Here's how the part is built. I have some questions about the finished solid (model axes, mm). A direction names the side the tool comes from. Round coordinates to 2 decimals unless told otherwise and drop trailing zeros. Loops run counter-clockwise (first coordinate to the right, second up) from the corner with the lowest first, then second, coordinate; pieces in that order, holes last. Notation, with made-up numbers: (-13.75, 32) -> (-3.75, 32) arc R37 cw to (-3.75, 71) -> close; hole circle Ø6 at (-16, 8.25). An arc over 180 degrees is marked (long way). One line per item, written item: value. Start each with the question number.
```python
from build123d import *

# Parameters (mm, degrees)
PAD_DEPTH    = 30
SKETCH001_R  = 3
POCKET_DEPTH = 5


with BuildPart() as part:
    # Sketch → Pad (new body)
    with BuildSketch(Plane.XY):
        Polygon((0, 0), (0, 53), (47.1, 53), (47.1, 50), (14, 50), (14, 0), (11, 0), (11, 48), (3, 48), (3, 0), align=None)
    extrude(amount=PAD_DEPTH)

    # Sketch001 (on Face2 of Pad) → Pocket (cut)
    with BuildSketch(Plane(origin=(0, 53, 0), x_dir=(-1, 0, 0), z_dir=(0, 1, 0))):
        with Locations((-32.1, 9)):
            Circle(SKETCH001_R)
        with Locations((-42.1, 25)):
            Circle(SKETCH001_R)
        with Locations((-42.1, 5)):
            Circle(SKETCH001_R)
        with Locations((-32.4, 21)):
            Circle(SKETCH001_R)
    extrude(amount=-POCKET_DEPTH, mode=Mode.SUBTRACT)


solid = part.part
```
Q1. I want a section at B-B on x = 42.1. Please give me the cut outline in (y, z), plus the area to 3 significant figures.
Q2. I want a section at D-D on x = 31. Please give me the cut outline in (y, z), plus the area to 3 significant figures.
Q3. If we mould it in two halves opening along X, with no side actions, what happens to faces 4 (the flat face through (13, 0, 15)), 5 (the flat face through (14, 25, 15)), 6 (the cylindrical face through (35.1, 51.5, 9.1))? For each: released by +X, released by -X, zero draft, split by the parting line, or undercut.
Q4. I want a section at A-A on y = 44. Please give me the cut outline in (x, z).
Q5. If I drill on line 1 along Z through (x, y) = (42.1, 52); line 2 along Z through (x, y) = (32.4, 51.3); line 3 along X through (y, z) = (39, 27.5), over which ranges is the centre line in solid material (lowest first)?
Q6. Will these pins go through, and if not, where does the flat tip stop? P1, Ø4, axis at y = 29, z = 10, coming from the +X side; P2, Ø7, axis at x = 42.1, z = 5, coming from the -Y side; P3, Ø5, axis at x = 32.1, z = 9, coming from the -Y side; P4, Ø2.5, axis at x = 7.5, z = 10.5, coming from the -Y side.
Q7. I want a section at C-C on z = 5. Please give me the cut outline in (x, y).
Q8. Which directions (+Z, -Z, +X, -X, +Y, -Y) give clear straight access to the entire face, cutting with the end or side of a thin tool? Please do faces 1 (the flat face through (31, 50, 15)), 2 (the cylindrical face through (29.63, 51.52, 19.85)), 3 (the flat face through (3, 24, 15)).
Answers below:
1. outline: (50, 0) -> (53, 0) -> (53, 2) -> (50, 2) -> close; (50, 8) -> (53, 8) -> (53, 22) -> (50, 22) -> close; (50, 28) -> (53, 28) -> (53, 30) -> (50, 30) -> close
1. area: 54.0 mm^2
2. outline: (50, 0) -> (53, 0) -> (53, 6.21) -> (50, 6.21) -> close; (50, 11.79) -> (53, 11.79) -> (53, 18.35) -> (50, 18.35) -> close; (50, 23.65) -> (53, 23.65) -> (53, 30) -> (50, 30) -> close
2. area: 57.3 mm^2
3. face 4: zero draft
3. face 5: released by +X
3. face 6: undercut
4. outline: (0, 0) -> (3, 0) -> (3, 30) -> (0, 30) -> close; (11, 0) -> (14, 0) -> (14, 30) -> (11, 30) -> close
5. line 1: z = 0 to 2, 8 to 22, 28 to 30
5. line 2: z = 0 to 6.02, 11.98 to 18, 24 to 30
5. line 3: x = 0 to 3, 11 to 14
6. P1: stops at x = 14
6. P2: stops at y = 50
6. P3: passes through
6. P4: stops at y = 48
7. outline: (0, 0) -> (3, 0) -> (3, 48) -> (11, 48) -> (11, 0) -> (14, 0) -> (14, 50) -> (39.1, 50) -> (39.1, 53) -> (0, 53) -> close; (45.1, 50) -> (47.1, 50) -> (47.1, 53) -> (45.1, 53) -> close
8. face 1: +Z, -Z, +X, -Y
8. face 2: +Y, -Y
8. face 3: +Z, -Z, -Y
